from build123d import *

# Parameters (mm, degrees)
DODANIE_WYCI_GNI_CIE1_DEPTH = 80


with BuildPart() as part:
    # Szkic1 → Dodanie-wyciągnięcie1 (new body)
    with BuildSketch(Plane.XY):
        Polygon((-30.708202586, 0), (30.708202586, 0), (28.873930311, 35), (27.873930311, 35), (26.294482101, 4.862332812), (25.294482101, 4.862332812), (23.715033891, 35), (22.715033891, 35), (21.135585681, 4.862332812), (20.135585681, 4.862332812), (18.556137471, 35), (17.556137471, 35), (15.976689261, 4.862332812), (14.976689261, 4.862332812), (13.39724105, 35), (12.39724105, 35), (10.81779284, 4.862332812), (9.81779284, 4.862332812), (8.23834463, 35), (7.23834463, 35), (5.65889642, 4.862332812), (4.65889642, 4.862332812), (3.07944821, 35), (2.07944821, 35), (0.5, 4.862332812), (-0.5, 4.862332812), (-2.07944821, 35), (-3.07944821, 35), (-4.65889642, 4.862332812), (-5.65889642, 4.862332812), (-7.23834463, 35), (-8.23834463, 35), (-9.81779284, 4.862332812), (-10.81779284, 4.862332812), (-12.39724105, 35), (-13.39724105, 35), (-14.976689261, 4.862332812), (-15.976689261, 4.862332812), (-17.556137471, 35), (-18.556137471, 35), (-20.135585681, 4.862332812), (-21.135585681, 4.862332812), (-22.715033891, 35), (-23.715033891, 35), (-25.294482101, 4.862332812), (-26.294482101, 4.862332812), (-27.873930311, 35), (-28.873930311, 35), (-30.453378521, 4.862332812), align=None)
    extrude(amount=-DODANIE_WYCI_GNI_CIE1_DEPTH)


solid = part.part
Read the model definition and answer for the solid it produces. Units are mm, in the model's axes. A direction names the side the tool comes from. Give positions to 0.01 mm unless a question says otherwise; leave off trailing zeros. Write each question's results on one line, items separated by ' | '.
1. Straight lines are drawn through the part: line 1 (Y direction, x = 20.5, z = -22); line 2 (X direction, y = 2, z = -34). For each, find the intervals that lie inside material, in ascending order. Write a range as [from, to].
Values:
line 1: y = [0, 4.86] | line 2: x = [-30.6, 30.6]
2. Section A-A on y = 24.5 is taken. State how many separate pieces and enclosed holes the cut face has, plus the area to 3 significant figures.
Values:
separate pieces: 12 | enclosed holes: 0 | area: 2,020 mm^2
3. The mould has two halves that part along X. Classify faces 1 (the face through (29.8, 17.3, -39.4)), 2 (the face through (11.62, 20.14, -39.44)), 3 (the face through (0, 0, -39)), 4 (the face through (3.88, 19.72, -39.44)): pulls with the +X half, pulls with the -X half, needs draft (parallel to the pull), parting line crosses it, or undercut.
Values:
face 1: pulls with the +X half | face 2: undercut | face 3: needs draft | face 4: undercut
4. Given pin 1 (1.5 mm diameter, centred on y = 28, z = -35, fed in from -X); pin 2 (12 mm diameter, centred on y = 19.5, z = -60.5, fed in from +X); pin 3 (10 mm diameter, centred on y = 16.5, z = -38.5, fed in from +X), each flat-ended and moving along its own axis, determine where each tip first touches the part or whether it passes through.
Values:
pin 1: stops at x = -29.28 | pin 2: stops at x = 30 | pin 3: stops at x = 30.11
5. A tool of negligible diameter and unlimited length cuts with its end or side. For faces 5 (the face through (-19.335, 20.142, -39.44)), 6 (the face through (-7, 14, 0)), from which of +Z, -Z, +X, -X, +Y, -Y can it reach the whole face along a straight path? Write none if from no direction.
Values:
face 5: +Z, -Z, +Y | face 6: +Z, +X, -X, +Y, -Y
